For this review, take the finished solid that the model builds, in its own axes (mm). A direction names the side the tool comes from. Coordinates: 2 decimals unless noted, no trailing zeros. Order: outer loops, then holes, each group sorted by start corner. A loop starts at its lowest first (then second) coordinate and runs counter-clockwise, first axis right, second up. Notation, with made-up numbers: (16.5, 66.5) -> (49.5, 66.5) arc R21 ccw to (49.5, 90.5) -> close; hole circle Ø2 at (74, 13.25). An arc over 180 degrees is marked (long way). Return JSON: item names as keys, results as strings. Group by question number.
Item 1: Take a section at A-A (x = 20). Write out the cut boundary in (y, z), then the cut area to 3 significant figures.
Item 2: Take a section at B-B (y = 18). Write out the cut boundary in (x, z).
Item 3: For line 1 along Y through (x, z) = (17, 2.05); line 2 along X through (y, z) = (18, 0.25); line 3 along X through (y, z) = (36.5, 0.25), list the stretches that pass through material, from the lowest coordinate up.
Item 4: Take a section at C-C (y = 37). Write out the cut boundary in (x, z).
Item 5: Machinability: for faces 4 (the flat face through (0, 62.49, 2)), 5 (the flat face through (0, 56.2, 2)), which of the approach directions +Z, -Z, +X, -X, +Y, -Y give a long, thin tool a straight path to every point of the face, cutting with its end or side? Answer none if there is none.
Item 6: Take a section at D-D (z = 2.7). Write out the cut boundary in (x, y), then the cut area to 3 significant figures.
Item 7: Draft analysis for pull direction Y (two halves, no side actions). For faces 1 (the flat face through (0, 10.268, 2)), 2 (the cylindrical face through (-37.667, 61.777, 1.568)), 3 (the flat face through (38.39, 37, 2)), state which applies: +Y half, -Y half, draft (parallel to the pull), parting line (faces both ways), or undercut.
```python
from build123d import *

# Parameters (mm, degrees)
SKETCH1_R   = 4.5
SKETCH1_W   = 50.090098238
SKETCH1_H   = 45.932062837
BEZEL_DEPTH = 3.18


with BuildPart() as part:
    # Sketch1 → Bezel (new body)
    with BuildSketch(Plane.XY):
        with BuildLine():
            Line((-35.919151108, 4.418014642), (29.997375098, 4.418014642))
            ThreePointArc((29.997375098, 4.418014642), (35.990372343, 7.41277043), (38.389642662, 13.668014642))
            Line((38.389642662, 13.668014642), (38.389642662, 59.990077479))
            ThreePointArc((38.389642662, 59.990077479), (37.657409615, 61.757844432), (35.889642662, 62.490077479))
            Line((35.889642662, 62.490077479), (-35.919151108, 62.490077479))
            ThreePointArc((-35.919151108, 62.490077479), (-37.686918061, 61.757844432), (-38.419151108, 59.990077479))
            Line((-38.419151108, 59.990077479), (-38.419151108, 6.918014642))
            ThreePointArc((-38.419151108, 6.918014642), (-37.686918061, 5.150247689), (-35.919151108, 4.418014642))
        make_face()
        with Locations(Location((-32.845865367, 40.325993685, 0), (0, 0, 180))):
            Circle(SKETCH1_R, mode=Mode.SUBTRACT)
        with Locations((-0.014754223, 33.23404606)):
            Rectangle(SKETCH1_W, SKETCH1_H, mode=Mode.SUBTRACT)
    extrude(amount=BEZEL_DEPTH)


solid = part.part
```
Findings below:
{
 "1": {"outline": "(4.42, 0) -> (10.27, 0) -> (10.27, 3.18) -> (4.42, 3.18) -> close; (56.2, 0) -> (62.49, 0) -> (62.49, 3.18) -> (56.2, 3.18) -> close", "area": "38.6 mm2"},
 "2": {"outline": "(-38.42, 0) -> (-25.06, 0) -> (-25.06, 3.18) -> (-38.42, 3.18) -> close; (25.03, 0) -> (38.39, 0) -> (38.39, 3.18) -> (25.03, 3.18) -> close"},
 "3": {"line 1": "y = 4.42 to 10.27, 56.2 to 62.49", "line 2": "x = -38.42 to -25.06, 25.03 to 38.39", "line 3": "x = -38.42 to -35.21, -30.48 to -25.06, 25.03 to 38.39"},
 "4": {"outline": "(-38.42, 0) -> (-35.88, 0) -> (-35.88, 3.18) -> (-38.42, 3.18) -> close; (-29.81, 0) -> (-25.06, 0) -> (-25.06, 3.18) -> (-29.81, 3.18) -> close; (25.03, 0) -> (38.39, 0) -> (38.39, 3.18) -> (25.03, 3.18) -> close"},
 "5": {"face 4": "+Z, -Z, +X, -X, +Y", "face 5": "+Z, -Z"},
 "6": {"outline": "(-38.42, 6.92) arc R2.5 ccw to (-35.92, 4.42) -> (30, 4.42) arc R9.25 ccw to (38.39, 13.67) -> (38.39, 59.99) arc R2.5 ccw to (35.89, 62.49) -> (-35.92, 62.49) arc R2.5 ccw to (-38.42, 59.99) -> close; hole circle Ø9 at (-32.85, 40.33); hole (-25.06, 10.27) -> (25.03, 10.27) -> (25.03, 56.2) -> (-25.06, 56.2) -> close", "area": "2,070 mm2"},
 "7": {"face 1": "undercut", "face 2": "+Y half", "face 3": "draft"}
}
